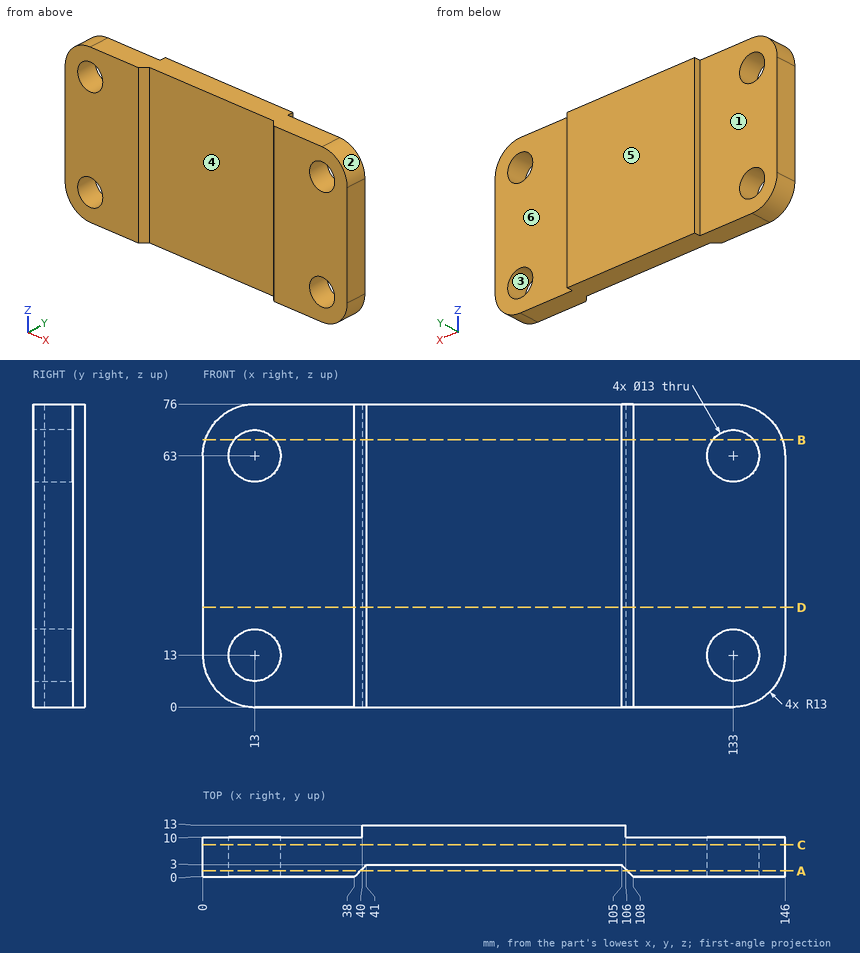
Here's the drawing with two shaded views (mm, measured from the low corner). I have some questions. A direction names the side the tool comes from. Give positions to 0.01 mm unless a question says otherwise; leave off trailing zeros. Loops run counter-clockwise (first coordinate to the right, second up) from the corner with the lowest first, then second, coordinate; pieces in that order, holes last. Notation, with made-up numbers: (74.25, 89.5) - (122.25, 89.5) arc R18 ccw to (122.25, 116.5) - close; hole circle Ø3 at (42.5, 39.25). An arc over 180 degrees is marked (long way). Return JSON: item names as keys, results as strings.
1. I want a section at D-D on z = 25. Please give me the cut outline in (x, y), and give its area (3 significant figures).
Output values:
{"outline": "(0, 0) - (38, 0) - (41, 3) - (105, 3) - (108, 0) - (146, 0) - (146, 10) - (106, 10) - (106, 13) - (40, 13) - (40, 10) - (0, 10) - close", "area": "1,460 mm²"}
2. We'd pull the mould along Z, two halves only. Please class the marked faces 1, 2 and 3: +Z half, -Z half, draft (parallel to the pull), parting line (faces both ways), or undercut.
Output values:
{"face 1": "draft", "face 2": "+Z half", "face 3": "undercut"}
3. I want a section at C-C on y = 8. Please give me the cut outline in (x, z), and give its area (3 significant figures).
Output values:
{"outline": "(0, 13) arc R13 ccw to (13, 0) - (133, 0) arc R13 ccw to (146, 13) - (146, 63) arc R13 ccw to (133, 76) - (13, 76) arc R13 ccw to (0, 63) - close; hole circle Ø13 at (13, 13); hole circle Ø13 at (13, 63); hole circle Ø13 at (133, 13); hole circle Ø13 at (133, 63)", "area": "10,400 mm²"}
4. I want a section at A-A on y = 1.5. Please give me the cut outline in (x, z).
Output values:
{"outline": "(0, 13) arc R13 ccw to (13, 0) - (39.5, 0) - (39.5, 76) - (13, 76) arc R13 ccw to (0, 63) - close; (106.5, 0) - (133, 0) arc R13 ccw to (146, 13) - (146, 63) arc R13 ccw to (133, 76) - (106.5, 76) - close; hole circle Ø13 at (13, 13); hole circle Ø13 at (13, 63); hole circle Ø13 at (133, 13); hole circle Ø13 at (133, 63)"}
5. I'm going to push flat-ended pins straight in: pin 1 Ø19 at (x, z) = (70.5, 55.5) entering from -Y; pin 2 Ø11.5 at (x, z) = (13, 13) entering from -Y; pin 3 Ø1.5 at (y, z) = (12, 20) entering from -X; pin 4 Ø1.5 at (y, z) = (12, 41) entering from +X. Where does each tip first touch, or does it pass through?
Output values:
{"pin 1": "stops at y = 3", "pin 2": "passes through", "pin 3": "stops at x = 40", "pin 4": "stops at x = 106"}
6. For the marked faces 4, 5 and 6, which set-ups out of +Z, -Z, +X, -X, +Y, -Y let a thin tool reach every point of the face, with its end or its side?
Output values:
{"face 4": "+Z, -Z, -Y", "face 5": "+Z, -Z, +X, -X, +Y", "face 6": "+Z, -Z, +X, +Y"}
7. If I drill on line 1 (X direction, y = 7.5, z = 63); line 2 (Z direction, x = 11, y = 3); line 3 (Y direction, x = 33.5, z = 9), over which ranges is the centre line in solid material (lowest first)?
Output values:
{"line 1": "x = 0 to 6.5, 19.5 to 126.5, 139.5 to 146", "line 2": "z = 0.15 to 6.82, 19.18 to 56.82, 69.18 to 75.85", "line 3": "y = 0 to 10"}
8. I want a section at B-B on z = 67. Please give me the cut outline in (x, y), and give its area (3 significant figures).
Output values:
{"outline": "(0.63, 0) - (7.88, 0) - (7.88, 10) - (0.63, 10) - close; (18.12, 0) - (38, 0) - (41, 3) - (105, 3) - (108, 0) - (127.88, 0) - (127.88, 10) - (106, 10) - (106, 13) - (40, 13) - (40, 10) - (18.12, 10) - close; (138.12, 0) - (145.37, 0) - (145.37, 10) - (138.12, 10) - close", "area": "1,240 mm²"}
